Can you work these out from the drawing? Everything is in mm from the part's minimum corner. A direction names the side the tool comes from. Give positions to 0.01 mm unless a question says otherwise; leave off trailing zeros. Write each loop counter-clockwise with the first axis right and the second up, starting at its lowest first coordinate (ties: lowest second). Pieces come first, ordered by that corner, then holes. Notation, with made-up numbers: (31, 72.5) - (76, 72.5) arc R27 ccw to (76, 94.5) - close; hole circle Ø5 at (34.5, 22.5). An arc over 180 degrees is marked (long way). Answer in a Markdown table with one row per item.
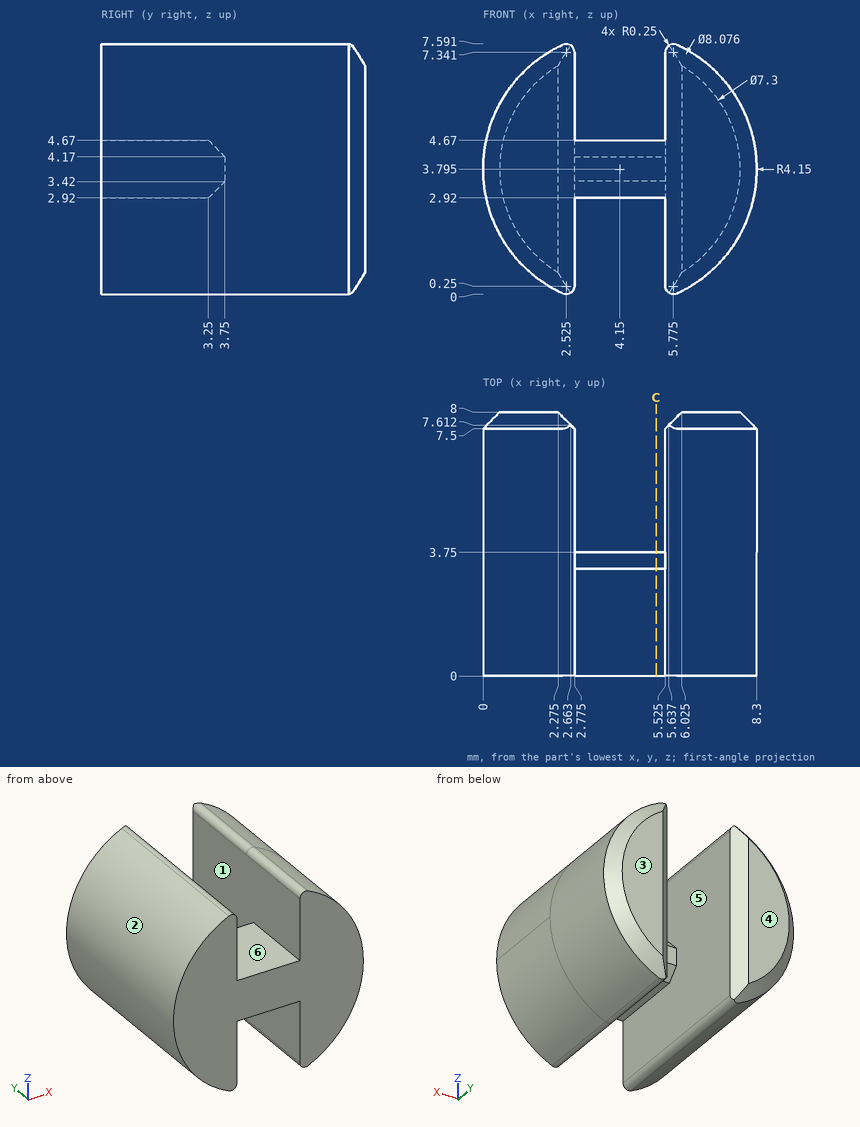
1) Will these pins go through, and if not, where does the flat tip stop? P1, Ø1.5, axis at x = 4.5, y = 5, coming from the +Z side; P2, Ø1.5, axis at y = 3.5, z = 1, coming from the -X side; P3, Ø1, axis at y = 1.5, z = 6.5, coming from the -X side (1 decimal); P4, Ø4, axis at y = 3.5, z = 1, coming from the +X side.
Check values:
| item | result |
|---|---|
| P1 | passes through |
| P2 | stops at x = 0.54 |
| P3 | stops at x = 0.6 |
| P4 | stops at x = 8.22 |
2) We'd pull the mould along X, two halves only. Please class the marked faces 1, 2 and 3: +X half, -X half, draft (parallel to the pull), parting line (faces both ways), or undercut.
Check values:
| item | result |
|---|---|
| face 1 | undercut |
| face 2 | -X half |
| face 3 | draft |
3) Imagine slicing it at C-C (x = 5.25). List the corners of the cut face in (y, z) for me.
Check values:
| item | result |
|---|---|
| outline | (0, 2.92) - (3.25, 2.92) - (3.75, 3.42) - (3.75, 4.17) - (3.25, 4.67) - (0, 4.67) - close |
4) If I drill on line 1 (X direction, y = 0.5, z = 1.5) (1 decimal); line 2 (X direction, y = 5.25, z = 3.75) (1 decimal); line 3 (Y direction, x = 3.75, z = 3.5), over which ranges is the centre line in solid material (lowest first)?
Check values:
| item | result |
|---|---|
| line 1 | x = 0.7 to 2.8, 5.5 to 7.6 |
| line 2 | x = 0 to 2.8, 5.5 to 8.3 |
| line 3 | y = 0 to 3.75 |
5) On a 3-axis mill with a long thin cutter (end or side, diameter ignored), from which of +Z, -Z, +X, -X, +Y, -Y can I reach the whole of each face in a straight line? I mean the marked faces 4, 5 and 6. Say none if no direction works.
Check values:
| item | result |
|---|---|
| face 4 | +Z, -Z, +X, -X, +Y |
| face 5 | +Y |
| face 6 | +Z, +Y, -Y |
